from build123d import *

# Parameters (mm, degrees)
BOSS_EXTRUDE1_DEPTH = 3.96875
SKETCH3_R           = 3.175
BOSS_EXTRUDE2_DEPTH = 57.15


with BuildPart() as part:
    # Sketch1 → Boss-Extrude1 (new body)
    with BuildSketch(Plane(origin=(0, 0, 0), x_dir=(1, 0, 0), z_dir=(0, 1, 0))):
        Polygon((6.415804866, 0), (3.207902433, 5.55625), (-3.207902433, 5.55625), (-6.415804866, 0), (-3.207902433, -5.55625), (3.207902433, -5.55625), align=None)
    extrude(amount=BOSS_EXTRUDE1_DEPTH)

    # Sketch2 → Cut-Revolve1 (revolve, cut)
    with BuildSketch(Plane.XY):
        with BuildLine():
            Line((6.415804866, 0.254), (6.415804866, 0))
            Line((6.415804866, 0), (5.592494081, 0))
            ThreePointArc((5.592494081, 0), (6.023294687, 0.064943068), (6.415804866, 0.254))
        make_face()
    revolve(axis=Axis((0, 0, 0), (0, 1, 0)), mode=Mode.SUBTRACT)

    # Sketch3 → Boss-Extrude2 (add)
    with BuildSketch(Plane(origin=(0, 0, 0), x_dir=(1, 0, 0), z_dir=(0, 1, 0))):
        Circle(SKETCH3_R)
    extrude(amount=BOSS_EXTRUDE2_DEPTH)


solid = part.part
Geometry check sheet. Reference: the model listing, model coordinates, mm. A direction names the side the tool comes from. Coordinates: 2 decimals unless noted, no trailing zeros. Loops run counter-clockwise (first coordinate to the right, second up) from the corner with the lowest first, then second, coordinate; pieces in that order, holes last. Notation, with made-up numbers: (-4.5, -30.5) - (27.5, -30.5) arc R11 cw to (27.5, -22.5) - close; hole circle Ø7 at (64.5, 44.25). An arc over 180 degrees is marked (long way). Use one line per item in the form item = value. Start each with the question number.
Item 1: Section check B-B, the plane y = 24. Enter the section's corners in (x, z) (3 decimals), and give its area (3 significant figures).
Item 2: Gauge pin test, flat ends, axial feed: pin 1 (2 mm diameter, centred on y = 29, z = 1.5, fed in from +X); pin 2 (1 mm diameter, centred on y = 8, z = -3, fed in from -X); pin 3 (1 mm diameter, centred on y = 41, z = 2, fed in from +X). Record the tip position at first contact, or that the pin passes through.
Item 3: Thickness scan on probe 1 along Y at (x, z) = (-3, 2.5); probe 2 along Z at (x, y) = (-0.25, 36.5); probe 3 along X at (y, z) = (54, 2.25). Record the ranges inside material, lowest first.
Item 4: Tool access check on faces 1 (the face through (-0.69, 30.19, 3.1)), 2 (the face through (0, 2, 5.556)). Record the directions out of +Z, -Z, +X, -X, +Y, -Y that give a thin tool (end or side, any length) a straight path to the whole face; none if there is none.
Item 5: Section check A-A, the plane x = 0. Enter the section's corners in (y, z) (3 decimals), and give its area (3 significant figures).
Computed:
q1.outline = circle Ø6.35 at (0, 0)
q1.area = 31.7 mm2
q2.pin_1 = 3.14
q2.pin_2 = -1.96
q2.pin_3 = 2.8
q3.probe_1 = 0 to 3.97
q3.probe_2 = -3.17 to 3.17
q3.probe_3 = -2.24 to 2.24
q4.face_1 = +Y
q4.face_2 = +Z, +X, -X, +Y, -Y
q5.outline = (0, -5.556) - (3.969, -5.556) - (3.969, -3.175) - (57.15, -3.175) - (57.15, 3.175) - (3.969, 3.175) - (3.969, 5.556) - (0, 5.556) - close
q5.area = 382 mm2
